```python
from build123d import *

# Parameters (mm, degrees)
F1_DEPTH  = 121.92
F3_DEPTH  = 282.829943269
F4_W      = 137.4469886072
F4_H      = 60.96
F4_H_2    = 25.5973618478
F5_DEPTH  = 1232.2696308848
F6_W      = 35.4420293589
F6_H      = 60.96
F5_FACE_W = 35.4420293589
F5_FACE_H = 25.5973618478
F7_DEPTH  = 131.2443939971


with BuildPart() as f1:
    # F0 (on Top) → F1 (new body)
    with BuildSketch(Plane.XY):
        with BuildLine():
            Line((0, 1557.528), (0, 97.2259938717))
            Line((0, 97.2259938717), (97.1533879638, 0))
            ThreePointArc((97.1533879638, 0), (161.1479027225, 77.3205102489), (200.2349644899, 169.7648763657))
            Line((200.2349644899, 169.7648763657), (240.7975746215, 169.7648763657))
            ThreePointArc((240.7975746215, 169.7648763657), (255.122674282, 887.0230394729), (0, 1557.528))
        make_face()
    extrude(amount=F1_DEPTH)

    # F2 (on face) → F3 (cut, through all)
    with BuildSketch(Plane(origin=(0, 0, 0), x_dir=(0, -1, 0), z_dir=(-1, 0, 0))):
        with BuildLine():
            Line((-97.2259938717, 121.92), (-1557.528, 121.92))
            ThreePointArc((-1557.528, 121.92), (-828.4837557125, 64.9274989858), (-97.2259938717, 60.96))
            Line((-97.2259938717, 60.96), (-97.2259938717, 121.92))
        make_face()
        with BuildLine():
            ThreePointArc((-97.2259938717, 25.5973618478), (-830.4601765145, 27.0160520849), (-1557.528, 121.92))
            Line((-1557.528, 121.92), (-1557.528, 0))
            Line((-1557.528, 0), (-97.2259938717, 0))
            Line((-97.2259938717, 0), (-97.2259938717, 25.5973618478))
        make_face()
    extrude(amount=-F3_DEPTH, mode=Mode.SUBTRACT)

    # F4 (on face) → F5 (cut, through all)
    with BuildSketch(Plane(origin=(48.6129833707, 48.5766804268, 0), x_dir=(0.7068426085, -0.7073708552, 0), z_dir=(-0.7073708552, -0.7068426085, 0))):
        with Locations((-0.0513401263, 91.44)):
            Rectangle(F4_W, F4_H)
        with Locations((-0.0513401263, 12.7986809239)):
            Rectangle(F4_W, F4_H_2)
    extrude(amount=-F5_DEPTH, mode=Mode.SUBTRACT)

    # F6 (on face) + F5_face (on face) → F7 (cut, through all)
    with BuildSketch(Plane(origin=(48.5404045931, -48.5766804268, 0), x_dir=(-0.7073708552, -0.7068426085, 0), z_dir=(-0.7068426085, 0.7073708552, 0))):
        with Locations((-86.4444898061, 91.44)):
            Rectangle(F6_W, F6_H)
    with BuildSketch(Plane(origin=(109.6887172721, 12.5259682421, 91.44), x_dir=(-0.7073708552, -0.7068426085, 0), z_dir=(-0.7068426085, 0.7073708552, 0))):
        with Locations((0, -78.6413190761)):
            Rectangle(F5_FACE_W, F5_FACE_H)
    extrude(amount=-F7_DEPTH, mode=Mode.SUBTRACT)

    # F8: F1 across face


with BuildPart() as f1_1:
    add(f1.part)
    add(f1.part.mirror(Plane(origin=(0, 690.8470850267, 48.623085259), x_dir=(0, -1, 0), z_dir=(-1, 0, 0))))


solid = f1_1.part
```
The listing builds one solid part. Answer for the finished solid, in the listing's coordinates (mm). A direction names the side the tool comes from. Give positions to 0.01 mm unless a question says otherwise; leave off trailing zeros. Order: outer loops, then holes, each group sorted by start corner. A loop starts at its lowest first (then second) coordinate and runs counter-clockwise, first axis right, second up. Notation, with made-up numbers: (-3.75, -37) -> (44.25, -37) arc R24 cw to (44.25, -9) -> close; hole circle Ø8 at (3, 40.25). An arc over 180 degrees is marked (long way). Answer as a JSON object with one key per item and string values. Group by question number.
Item 1: Consider L1, parallel to Z at x = 36, y = 475; L2, parallel to Z at x = -188.5, y = 366; L3, parallel to X at y = 1077, z = 73.5. Determine where each line is inside the solid, lowest interval first. Write a range as from..to.
Item 2: The part is cut by section B-B on z = 98. Write down the section's boundary in (x, y).
Item 3: Determine the mould class of faces 1 (the flat face through (-145, 168, 25.597)), 2 (the cylindrical face through (160.414, 76.117, 43.031)), 3 (the flat face through (47.9, 49.29, 43.03)) for opening direction X: pulls with the +X half, pulls with the -X half, needs draft (parallel to the pull), parting line crosses it, or undercut.
Item 4: The part is cut by section C-C on y = 1264. Write down the section's boundary in (x, z), and give its area (3 significant figures).
Item 5: The part is cut by section A-A on x = -43. Write down the section's boundary in (y, z).
Item 6: A tool of negligible diameter and unlimited length cuts with its end or side. For faces 4 (the flat face through (164.701, 261.804, 21.471)), 5 (the flat face through (-164.701, 261.804, 21.471)), 6 (the flat face through (-47.9, 49.29, 43.03)), from which of +Z, -Z, +X, -X, +Y, -Y can it reach the whole face along a straight path? Write none if from no direction.
Item 7: The part is cut by section D-D on x = 57. Write down the section's boundary in (y, z).
Item 8: Flat-ended cylindrical pins translate along their axes: pin 1 (1 mm diameter, centred on x = -6, y = 1231, fed in from -Z); pin 2 (8 mm diameter, centred on x = 109.5, y = 1127.5, fed in from +Z); pin 3 (4 mm diameter, centred on x = 135.5, y = 777.5, fed in from -Z). Find the tip coordinate at first contact, or state that the pin passes through.
Result set:
{
 "1": {"L1": "14.62..56.38", "L2": "15.23..56.25", "L3": "-211.92..211.92"},
 "2": {"outline": "(-122.44, 1325.52) -> (122.44, 1325.52) arc R1881.95 ccw to (73.58, 1427.72) -> (-73.58, 1427.72) arc R1881.95 ccw to start"},
 "3": {"face 1": "needs draft", "face 2": "pulls with the +X half", "face 3": "undercut"},
 "4": {"outline": "(-148.31, 72.2) -> (148.31, 72.2) -> (148.31, 92.57) -> (-148.31, 92.57) -> close", "area": "6,040 mm²"},
 "5": {"outline": "(54.19, 25.6) -> (140.19, 25.6) -> (140.19, 23.09) arc R5738.54 ccw to (1484.62, 108.1) -> (1484.62, 113.82) arc R10076.16 cw to (97.23, 60.96) -> (54.19, 60.96) -> close"},
 "6": {"face 4": "-Z, +X, -Y", "face 5": "-Z, -X, -Y", "face 6": "+Z, -Z, -Y"},
 "7": {"outline": "(40.18, 25.6) -> (154.18, 25.6) -> (154.18, 22.35) arc R5738.54 ccw to (1459.15, 103.51) -> (1459.15, 111.11) arc R10076.16 cw to (97.23, 60.96) -> (40.18, 60.96) -> close"},
 "8": {"pin 1": "z = 67.52", "pin 2": "z = 82.15", "pin 3": "z = 23.66"}
}
